```python
from build123d import *

# Parameters (mm, degrees)
SKETCH1_R           = 7.5
SKETCH1_R_2         = 1.8
BOSS_EXTRUDE1_DEPTH = 5
CUT_EXTRUDE1_DEPTH  = 6


with BuildPart() as part:
    # Sketch1 → Boss-Extrude1 (new body)
    with BuildSketch(Plane.XY):
        Polygon((-15, 30), (15, 30), (15, 25), (35, 25), (35, -25), (15, -25), (15, -30), (-15, -30), (-15, -25), (-35, -25), (-35, 25), (-15, 25), align=None)
        Circle(SKETCH1_R, mode=Mode.SUBTRACT)
        with Locations((4.7625, -8.248891971)):
            Circle(SKETCH1_R_2, mode=Mode.SUBTRACT)
        with Locations((-9.525, 0)):
            Circle(SKETCH1_R_2, mode=Mode.SUBTRACT)
        with Locations((4.7625, 8.248891971)):
            Circle(SKETCH1_R_2, mode=Mode.SUBTRACT)
    extrude(amount=BOSS_EXTRUDE1_DEPTH)

    # Sketch3 → Cut-Extrude1 (cut, through all)
    with BuildSketch(Plane.XY.offset(5)):
        Polygon((26.65, 25), (26.65, 21), (28.5, 21), (28.5, 18.8), (26.78859304, 18.8), (26.78859304, 16.8), (23.21140696, 16.8), (23.21140696, 18.8), (21.5, 18.8), (21.5, 21), (23.35, 21), (23.35, 25), align=None)
        Polygon((-23.35, 25), (-23.35, 21), (-21.5, 21), (-21.5, 18.8), (-23.21140696, 18.8), (-23.21140696, 16.8), (-26.78859304, 16.8), (-26.78859304, 18.8), (-28.5, 18.8), (-28.5, 21), (-26.65, 21), (-26.65, 25), align=None)
        Polygon((-26.65, -25), (-26.65, -21), (-28.5, -21), (-28.5, -18.8), (-26.78859304, -18.8), (-26.78859304, -16.8), (-23.21140696, -16.8), (-23.21140696, -18.8), (-21.5, -18.8), (-21.5, -21), (-23.35, -21), (-23.35, -25), align=None)
        Polygon((23.35, -25), (23.35, -21), (21.5, -21), (21.5, -18.8), (23.21140696, -18.8), (23.21140696, -16.8), (26.78859304, -16.8), (26.78859304, -18.8), (28.5, -18.8), (28.5, -21), (26.65, -21), (26.65, -25), align=None)
    extrude(amount=-CUT_EXTRUDE1_DEPTH, mode=Mode.SUBTRACT)


solid = part.part
```
The listing builds one solid part. Answer for the finished solid, in the listing's coordinates (mm). A direction names the side the tool comes from. Round coordinates to 2 decimals unless told otherwise and drop trailing zeros. Order: outer loops, then holes, each group sorted by start corner. A loop starts at its lowest first (then second) coordinate and runs counter-clockwise, first axis right, second up. Notation, with made-up numbers: (15.5, 12.5) -> (26.5, 12.5) arc R15 ccw to (26.5, 17.5) -> close; hole circle Ø5 at (35, 21). An arc over 180 degrees is marked (long way). Answer as CSV lines item,"result". Start each with the question number.
(1) Flat-ended cylindrical pins translate along their axes: pin 1 Ø0.9 at (x, z) = (-27.5, 3.5) entering from -Y; pin 2 Ø0.6 at (x, z) = (27.5, 1.5) entering from +Y; pin 3 Ø2.5 at (y, z) = (27, 3) entering from -X. Find the tip coordinate at first contact, or state that the pin passes through.
(2) The part is cut by section A-A (x = 0). Determine the outline of the cut face in (y, z).
(3) For a pull along Y with two mould halves and no side action, classify faces 1 (the face through (26.65, -23, 3)), 2 (the face through (23.211, -18, 3)), 3 (the face through (-31, 25, 2)) as +Y half, -Y half, draft (parallel to the pull), parting line (faces both ways), or undercut.
(4) The part is cut by section D-D (z = 3.3). Count the separate pieces of the cut face and the enclosed holes in it, then the cut area to 3 significant figures.
(5) A tool of negligible diameter and unlimited length cuts with its end or side. For faces 4 (the face through (-15, 27, 2)), 5 (the face through (31, -25, 2)), 6 (the face through (-23.211, 18, 3)), 7 (the face through (-26.65, 23, 3)), from which of +Z, -Z, +X, -X, +Y, -Y can it reach the whole face along a straight path? Write none if from no direction.
(6) Find the intervals of material crossed by probe 1 along X at (y, z) = (17.5, 3.35); probe 2 along Y at (x, z) = (6, 4.5); probe 3 along Y at (x, z) = (0, 1.6), in increasing order. Write a range as from..to.
(7) The part is cut by section C-C (x = -17.5). Determine the outline of the cut face in (y, z).
(8) The part is cut by section B-B (y = 0). Determine the outline of the cut face in (x, z) (3 decimals).
Evaluation:
1,pin 1,"y = -25"
1,pin 2,"y = 25"
1,pin 3,"x = -15"
2,outline,"(-30, 0) -> (-7.5, 0) -> (-7.5, 5) -> (-30, 5) -> close; (7.5, 0) -> (30, 0) -> (30, 5) -> (7.5, 5) -> close"
3,face 1,"draft"
3,face 2,"undercut"
3,face 3,"+Y half"
4,separate pieces,"1"
4,enclosed holes,"4"
4,area,"3,450 mm²"
5,face 4,"+Z, -Z, -X, +Y"
5,face 5,"+Z, -Z, +X, -Y"
5,face 6,"+Z, -Z"
5,face 7,"+Z, -Z, +Y"
6,probe 1,"-35..-26.79, -23.21..23.21, 26.79..35"
6,probe 2,"-30..-9.56, -6.94..-4.5, 4.5..6.94, 9.56..30"
6,probe 3,"-30..-7.5, 7.5..30"
7,outline,"(-25, 0) -> (25, 0) -> (25, 5) -> (-25, 5) -> close"
8,outline,"(-35, 0) -> (-11.325, 0) -> (-11.325, 5) -> (-35, 5) -> close; (-7.725, 0) -> (-7.5, 0) -> (-7.5, 5) -> (-7.725, 5) -> close; (7.5, 0) -> (35, 0) -> (35, 5) -> (7.5, 5) -> close"
